Geometry check sheet. Reference: the model listing, model coordinates, mm. Face numbers are marked on the shaded views. Give positions to 0.01 mm unless a question says otherwise; leave off trailing zeros. Loops run counter-clockwise (first coordinate to the right, second up) from the corner with the lowest first, then second, coordinate; pieces in that order, holes last. Notation, with made-up numbers: (22, 40.5) -> (76, 40.5) arc R34 ccw to (76, 78.5) -> close; hole circle Ø3 at (40, 26). An arc over 180 degrees is marked (long way). Answer as a JSON object with one key per item and string values.
from build123d import *

# Parameters (mm, degrees)
SKETCH1_W           = 98.425
SKETCH1_H           = 57.15
BOSS_EXTRUDE1_DEPTH = 25.4
SKETCH2_W           = 5.08
SKETCH2_H           = 45.72
BOSS_EXTRUDE2_DEPTH = 0.762
FILLET1_R           = 9.525
SKETCH3_W           = 7.14375
SKETCH3_H           = 14.2875
CUT_EXTRUDE1_DEPTH  = 1.27
SKETCH4_R           = 3.175
SKETCH4_W           = 12.7
SKETCH4_H           = 11.1125
CUT_EXTRUDE2_DEPTH  = 1.27


with BuildPart() as part:
    # Sketch1 → Boss-Extrude1 (new body)
    with BuildSketch(Plane(origin=(0, 0, 0), x_dir=(1, 0, 0), z_dir=(0, 1, 0))):
        Rectangle(SKETCH1_W, SKETCH1_H)
    extrude(amount=BOSS_EXTRUDE1_DEPTH)

    # Sketch2 → Boss-Extrude2 (add)
    with BuildSketch(Plane.XZ):
        with Locations((-40.3225, 0)):
            Rectangle(SKETCH2_W, SKETCH2_H)
        with Locations((40.3225, 0)):
            Rectangle(SKETCH2_W, SKETCH2_H)
    extrude(amount=BOSS_EXTRUDE2_DEPTH)

    # Fillet1
    fillet1_edges = [part.edges().sort_by_distance(p)[0] for p in [
        (-49.2125, 12.7, -28.575),
        (49.2125, 12.7, -28.575),
        (49.2125, 12.7, 28.575),
        (-49.2125, 12.7, 28.575),
    ]]
    fillet(fillet1_edges, radius=FILLET1_R)

    # Sketch3 → Cut-Extrude1 (cut)
    with BuildSketch(Plane(origin=(0, 0, -28.575), x_dir=(-1, 0, 0), z_dir=(0, 0, -1))):
        with Locations((-34.528125, 15.08125)):
            Rectangle(SKETCH3_W, SKETCH3_H)
        with Locations((-23.01875, 15.08125)):
            Rectangle(SKETCH3_W, SKETCH3_H)
        with Locations((-11.509375, 15.08125)):
            Rectangle(SKETCH3_W, SKETCH3_H)
        with Locations((0, 15.08125)):
            Rectangle(SKETCH3_W, SKETCH3_H)
        with Locations((11.509375, 15.08125)):
            Rectangle(SKETCH3_W, SKETCH3_H)
        with Locations((23.01875, 15.08125)):
            Rectangle(SKETCH3_W, SKETCH3_H)
        with Locations((34.528125, 15.08125)):
            Rectangle(SKETCH3_W, SKETCH3_H)
    extrude(amount=-CUT_EXTRUDE1_DEPTH, mode=Mode.SUBTRACT)

    # Sketch4 → Cut-Extrude2 (cut)
    with BuildSketch(Plane.XY.offset(28.575)):
        with Locations((-32.54375, 12.7)):
            Circle(SKETCH4_R)
        with Locations((-15.08125, 13.49375)):
            Rectangle(SKETCH4_W, SKETCH4_H)
    extrude(amount=-CUT_EXTRUDE2_DEPTH, mode=Mode.SUBTRACT)


solid = part.part
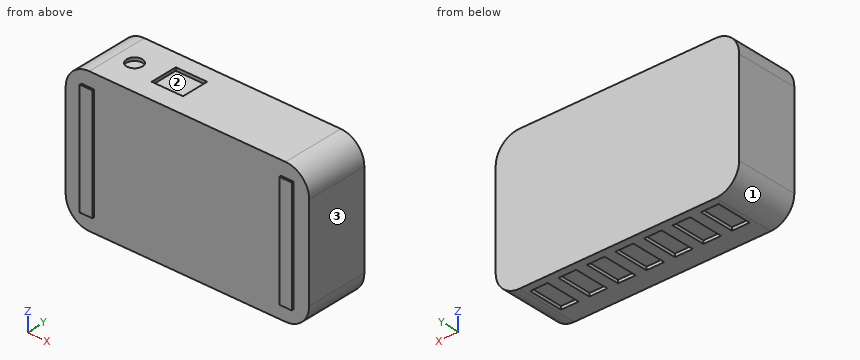
1) Section check A-A on x = -25.5. Record the cut outline in (y, z) (1 decimal).
Geometry check:
{"outline": "(0, -28.6) -> (7.9, -28.6) -> (7.9, -27.3) -> (22.2, -27.3) -> (22.2, -28.6) -> (25.4, -28.6) -> (25.4, 28.6) -> (0, 28.6) -> close"}
2) Material ranges on line 1 along Y through (x, z) = (22, 15); line 2 along Z through (x, y) = (-15.5, 15) (3 decimals); line 3 along Z through (x, y) = (-22.5, 22) (3 decimals), recorded low to high. Write a range as from..to.
Geometry check:
{"line 1": "y = 0..25.4", "line 2": "z = -28.575..27.305", "line 3": "z = -27.305..28.575"}
3) Section check B-B on z = -15. Record the cut outline in (x, y).
Geometry check:
{"outline": "(-49.21, 0) -> (-42.86, 0) -> (-42.86, -0.76) -> (-37.78, -0.76) -> (-37.78, 0) -> (37.78, 0) -> (37.78, -0.76) -> (42.86, -0.76) -> (42.86, 0) -> (49.21, 0) -> (49.21, 25.4) -> (-49.21, 25.4) -> close"}
4) Draft check along X on the marked faces 1, 2 and 3. Enter one of: pulls with the +X half, pulls with the -X half, needs draft (parallel to the pull), parting line crosses it, or undercut.
Geometry check:
{"face 1": "pulls with the -X half", "face 2": "undercut", "face 3": "pulls with the +X half"}
5) Depth check by flat-ended pin: P1, Ø3, axis at x = 21.5, y = 19, coming from the -Z side (3 decimals); P2, Ø1, axis at x = -19, y = 10, coming from the +Z side (3 decimals); P3, Ø1, axis at x = 20.5, z = -16.5, coming from the -Y side. Enter the tip coordinate at first touch or a pass-through.
Geometry check:
{"P1": "stops at z = -27.305", "P2": "stops at z = 27.305", "P3": "stops at y = 0"}
